The listing builds one solid part. Answer for the finished solid, in the listing's coordinates (mm). Give positions to 0.01 mm unless a question says otherwise; leave off trailing zeros. Order: outer loops, then holes, each group sorted by start corner. A loop starts at its lowest first (then second) coordinate and runs counter-clockwise, first axis right, second up. Notation, with made-up numbers: (35, 57.5) - (86, 57.5) arc R16 cw to (86, 62.5) - close; hole circle Ø9 at (53.25, 60.25). An arc over 180 degrees is marked (long way). Answer as CSV lines item,"result". Start each with the question number.
1. Section A-A on y = 11 is taken. Give the vertices of the cut face in (x, z).
2. Consider line 1 along X through (y, z) = (0, -0.55); line 2 along X through (y, z) = (-9, 0.2); line 3 along Y through (x, z) = (-1, 0.2). Determine where each line is inside the solid, lowest interval first. Write a range as [from, to].
3. Section B-B on x = 4 is taken. Give the vertices of the cut face in (y, z).
4. Flat-ended cylindrical pins translate along their axes: pin 1 (14 mm diameter, centred on x = -6, y = -10.5, fed in from -Z); pin 2 (0.5 mm diameter, centred on y = -8, z = 0.5, fed in from +X); pin 3 (3 mm diameter, centred on x = -15, y = 14.5, fed in from -Z); pin 4 (0.8 mm diameter, centred on y = -1, z = -0.5, fed in from +X). Find the tip coordinate at first contact, or state that the pin passes through.
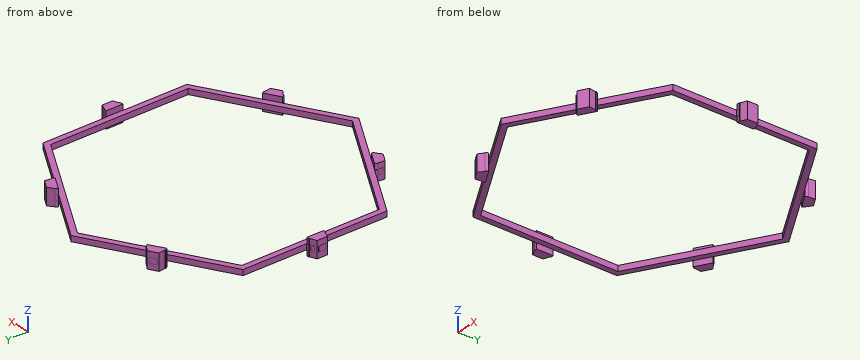
from build123d import *

# Parameters (mm, degrees)
BOSS_EXTRUDE1_DEPTH      = 1
BOSS_EXTRUDE2_DEPTH      = 1
BOSS_EXTRUDE2_DEPTH_BACK = 2


with BuildPart() as part:
    # Sketch1 → Boss-Extrude1 (new body)
    with BuildSketch(Plane.XY):
        with BuildLine():
            Line((22.397016434, 12.952378094), (12.476954775, 18.679728363))
            Line((12.476954775, 18.679728363), (12.726954775, 19.112741065))
            Line((12.726954775, 19.112741065), (12.516198987, 19.234420976))
            ThreePointArc((12.516198987, 19.234420976), (12.68450037, 19.874654921), (12.504090028, 20.511582679))
            Line((12.504090028, 20.511582679), (11.404603705, 21.146371403))
            ThreePointArc((11.404603705, 21.146371403), (10.775926893, 20.968706558), (10.316076863, 20.504662076))
            Line((10.316076863, 20.504662076), (10.128878563, 20.612741065))
            Line((10.128878563, 20.612741065), (9.878878563, 20.179728363))
            Line((9.878878563, 20.179728363), (-0.03711231, 25.904728363))
            Line((-0.03711231, 25.904728363), (-9.957173969, 20.177378094))
            Line((-9.957173969, 20.177378094), (-10.207173969, 20.610390796))
            Line((-10.207173969, 20.610390796), (-10.417929757, 20.488710885))
            ThreePointArc((-10.417929757, 20.488710885), (-10.888237926, 20.954581131), (-11.530038716, 21.116805071))
            Line((-11.530038716, 21.116805071), (-12.629525039, 20.482016346))
            ThreePointArc((-12.629525039, 20.482016346), (-12.790001175, 19.848733833), (-12.618051881, 19.218469784))
            Line((-12.618051881, 19.218469784), (-12.80525018, 19.110390796))
            Line((-12.80525018, 19.110390796), (-12.55525018, 18.677378094))
            Line((-12.55525018, 18.677378094), (-22.471241054, 12.952378094))
            Line((-22.471241054, 12.952378094), (-22.471241054, 1.901120277))
            Line((-22.471241054, 1.901120277), (-22.471241054, 1.497677556))
            Line((-22.471241054, 1.497677556), (-22.971241054, 1.497677556))
            Line((-22.971241054, 1.497677556), (-22.971241054, 1.254317734))
            ThreePointArc((-22.971241054, 1.254317734), (-23.609850606, 1.079954035), (-24.071241054, 0.605250217))
            Line((-24.071241054, 0.605250217), (-24.071241054, -0.664327233))
            ThreePointArc((-24.071241054, -0.664327233), (-23.603040378, -1.1199449), (-22.971241054, -1.286164467))
            Line((-22.971241054, -1.286164467), (-22.971241054, -1.502322444))
            Line((-22.971241054, -1.502322444), (-22.471241054, -1.502322444))
            Line((-22.471241054, -1.502322444), (-22.471241054, -1.596383326))
            Line((-22.471241054, -1.596383326), (-22.471241054, -12.952322444))
            Line((-22.471241054, -12.952322444), (-12.630090814, -18.634113185))
            Line((-12.630090814, -18.634113185), (-12.551179395, -18.679672714))
            Line((-12.551179395, -18.679672714), (-12.801179395, -19.112685416))
            Line((-12.801179395, -19.112685416), (-12.590423607, -19.234365326))
            ThreePointArc((-12.590423607, -19.234365326), (-12.758724991, -19.874599271), (-12.578314648, -20.511527029))
            Line((-12.578314648, -20.511527029), (-11.478828325, -21.146315754))
            ThreePointArc((-11.478828325, -21.146315754), (-10.850151513, -20.968650909), (-10.390301483, -20.504606427))
            Line((-10.390301483, -20.504606427), (-10.203103183, -20.612685416))
            Line((-10.203103183, -20.612685416), (-9.953103183, -20.179672714))
            Line((-9.953103183, -20.179672714), (-9.931256757, -20.192285754))
            Line((-9.931256757, -20.192285754), (-0.03711231, -25.904672714))
            Line((-0.03711231, -25.904672714), (9.790701603, -20.230581705))
            Line((9.790701603, -20.230581705), (9.882949349, -20.177322444))
            Line((9.882949349, -20.177322444), (10.132949349, -20.610335146))
            Line((10.132949349, -20.610335146), (10.343705136, -20.488655236))
            ThreePointArc((10.343705136, -20.488655236), (10.814013306, -20.954525482), (11.455814095, -21.116749421))
            Line((11.455814095, -21.116749421), (12.555300419, -20.481960696))
            ThreePointArc((12.555300419, -20.481960696), (12.715776555, -19.848678184), (12.543827261, -19.218414135))
            Line((12.543827261, -19.218414135), (12.73102556, -19.110335146))
            Line((12.73102556, -19.110335146), (12.48102556, -18.677322444))
            Line((12.48102556, -18.677322444), (12.549124227, -18.638005661))
            Line((12.549124227, -18.638005661), (22.397016434, -12.952322444))
            Line((22.397016434, -12.952322444), (22.397016434, -1.497621906))
            Line((22.397016434, -1.497621906), (22.897016434, -1.497621906))
            Line((22.897016434, -1.497621906), (22.897016434, -1.254262085))
            ThreePointArc((22.897016434, -1.254262085), (23.535625986, -1.079898386), (23.997016434, -0.605194567))
            Line((23.997016434, -0.605194567), (23.997016434, 0.664382882))
            ThreePointArc((23.997016434, 0.664382882), (23.528815758, 1.120000549), (22.897016434, 1.286220117))
            Line((22.897016434, 1.286220117), (22.897016434, 1.502378094))
            Line((22.897016434, 1.502378094), (22.397016434, 1.502378094))
            Line((22.397016434, 1.502378094), (22.397016434, 12.952378094))
        make_face()
        Polygon((21.397016434, 12.375027825), (-0.03711231, 24.750027825), (-21.471241054, 12.375027825), (-21.471241054, -12.374972175), (-0.03711231, -24.749972175), (21.397016434, -12.374972175), align=None, mode=Mode.SUBTRACT)
    extrude(amount=BOSS_EXTRUDE1_DEPTH)

    # Sketch2 → Boss-Extrude2 (add, two sides)
    with BuildSketch(Plane.XY.offset(1)) as boss_extrude2_sk:
        Polygon((-12.55525018, 18.677378094), (-9.957173969, 20.177378094), (-10.207173969, 20.610390796), (-10.312551863, 20.54955084), (-11.258459696, 21.268059485), (-12.867222828, 20.344781463), (-12.711651031, 19.16443029), (-12.80525018, 19.110390796), align=None)
        Polygon((11.185486168, 21.315732577), (12.789449955, 20.384141846), (12.640157133, 19.205707311), (12.745535027, 19.144867356), (12.495535027, 18.711854654), (9.897458815, 20.211854654), (10.147458815, 20.644867356), (10.241057965, 20.590827862), align=None)
        Polygon((24.052708996, 0.970951113), (24.047909651, -0.883917639), (22.952708996, -1.343843529), (22.952708996, -1.46552344), (22.452708996, -1.46552344), (22.452708996, 1.53447656), (22.952708996, 1.53447656), (22.952708996, 1.426397572), align=None)
        Polygon((12.867222828, -20.344781463), (11.258459696, -21.268059485), (10.312551863, -20.54955084), (10.207173969, -20.610390796), (9.957173969, -20.177378094), (12.55525018, -18.677378094), (12.80525018, -19.110390796), (12.711651031, -19.16443029), align=None)
        Polygon((-11.185486168, -21.315732577), (-12.789449955, -20.384141846), (-12.640157133, -19.205707311), (-12.745535027, -19.144867356), (-12.495535027, -18.711854654), (-9.897458815, -20.211854654), (-10.147458815, -20.644867356), (-10.241057965, -20.590827862), align=None)
        Polygon((-24.052708996, -0.970951113), (-24.047909651, 0.883917639), (-22.952708996, 1.343843529), (-22.952708996, 1.46552344), (-22.452708996, 1.46552344), (-22.452708996, -1.53447656), (-22.952708996, -1.53447656), (-22.952708996, -1.426397572), align=None)
    extrude(amount=BOSS_EXTRUDE2_DEPTH)
    extrude(boss_extrude2_sk.sketch, amount=-BOSS_EXTRUDE2_DEPTH_BACK)


solid = part.part
Checks:
1,outline,"(-22.47, 0) - (-21.47, 0) - (-21.47, 1) - (-22.47, 1) - close; (21.4, 0) - (22.4, 0) - (22.4, 1) - (21.4, 1) - close"
2,line 1,"x = [-24.05, -22.45], [22.45, 24.05]"
2,line 2,"x = [-22.47, -21.47], [21.4, 22.4]"
2,line 3,"y = [-25.35, -24.19], [24.19, 25.35]"
3,outline,"(-23.57, 0) - (-22.42, 0) - (-22.42, 1) - (-23.57, 1) - close; (22.42, 0) - (23.57, 0) - (23.57, 1) - (22.42, 1) - close"
4,pin 1,"passes through"
4,pin 2,"stops at x = 22.4"
4,pin 3,"stops at z = 0"
4,pin 4,"stops at x = 24.05"
